```python
from build123d import *

# Parameters (mm, degrees)
EXTRUDE010_DEPTH = 5
SKETCH010_R      = 2
EXTRUDE009_DEPTH = 5
SKETCH012_R      = 2.1
EXTRUDE011_DEPTH = 5


with BuildPart() as extrude010:
    # Sketch011 (on Face6 of Extrude009) → Extrude010 (new body)
    with BuildSketch(Plane(origin=(0, 64.406042, 20.6), x_dir=(-1, 0, 0), z_dir=(0, 1, 0))):
        with BuildLine():
            Line((-18.188271, 0), (-18.188271, 36.810456))
            ThreePointArc((-12.998727, 42), (-16.668289, 40.480018), (-18.188271, 36.810456))
            Line((-12.998727, 42), (37.622185, 42))
            ThreePointArc((42.811729, 36.810456), (41.291746, 40.480018), (37.622185, 42))
            Line((42.811729, 0), (42.811729, 36.810456))
            Line((-18.188271, 0), (42.811729, 0))
        make_face()
        with BuildLine():
            Line((-9.188271, 5), (-9.188271, 33.276052))
            ThreePointArc((-5.464323, 37), (-8.097552, 35.909281), (-9.188271, 33.276052))
            Line((-5.464323, 37), (30.08778, 37))
            ThreePointArc((33.811729, 33.276052), (32.721009, 35.909281), (30.08778, 37))
            Line((33.811729, 33.276052), (33.811729, 5))
            Line((-9.188271, 5), (33.811729, 5))
        make_face(mode=Mode.SUBTRACT)
    extrude(amount=-EXTRUDE010_DEPTH)


with BuildPart() as extrude009:
    # Sketch010 → Extrude009 (new body)
    with BuildSketch(Plane.XY):
        Polygon((11.188271, 48.406042), (11.188271, 59.406042), (-35.811729, 59.406042), (-35.811729, 48.406042), (-42.811729, 48.406042), (-42.811729, 64.406042), (18.188271, 64.406042), (18.188271, 48.406042), align=None)
        with Locations((-39.061729, 52.906042)):
            Circle(SKETCH010_R, mode=Mode.SUBTRACT)
        with Locations((14.438271, 52.906042)):
            Circle(SKETCH010_R, mode=Mode.SUBTRACT)
    extrude(amount=EXTRUDE009_DEPTH)


with BuildPart() as extrude009_1:
    # Extrude009 placement: moved
    add(extrude009.part.moved(Location((0, 0, 20.6))))


with BuildPart() as pcb_holder_fusion:
    # Sketch012 (on Face3 of Extrude010) → Extrude011 (new body)
    with BuildSketch(Plane.XY.offset(62.6)):
        with BuildLine():
            Line((-37.622185, 64.406042), (-37.622185, 58.771772))
            ThreePointArc((-37.622185, 58.771772), (-36.898048, 57.023553), (-35.149829, 56.299416))
            Line((-35.149829, 56.299416), (10.526371, 56.299416))
            ThreePointArc((10.526371, 56.299416), (12.274591, 57.023553), (12.998727, 58.771772))
            Line((12.998727, 64.406042), (12.998727, 58.771772))
            Line((-37.622185, 64.406042), (12.998727, 64.406042))
        make_face()
        with Locations((-27.801273, 59.699416)):
            Circle(SKETCH012_R, mode=Mode.SUBTRACT)
        with Locations((3.198727, 59.799416)):
            Circle(SKETCH012_R, mode=Mode.SUBTRACT)
    extrude(amount=-EXTRUDE011_DEPTH)


with BuildPart() as pcb_holder_fusion_1:
    # Extrude011 placement: moved
    add(pcb_holder_fusion.part.moved(Location((0, -5, 0))))

    # Fusion012: union Extrude010, Extrude009
    add(extrude010.part)
    add(extrude009_1.part)


solid = pcb_holder_fusion_1.part
```
Work out the finished part from the listing and answer in its coordinate system (mm). A direction names the side the tool comes from. Round coordinates to 2 decimals unless told otherwise and drop trailing zeros. Order: outer loops, then holes, each group sorted by start corner. A loop starts at its lowest first (then second) coordinate and runs counter-clockwise, first axis right, second up.
Q1. A tool of negligible diameter and unlimited length cuts with its end or side. For faces 1 (the flat face through (9.188, 62, 40)), 2 (the flat face through (12.999, 57, 60)), 3 (the flat face through (-39.3, 55.2, 25.6)), from which of +Z, -Z, +X, -X, +Y, -Y can it reach the whole face along a straight path? Write none if from no direction.
Solution:
face 1: +Y, -Y
face 2: +Z, +X, -Y
face 3: +X, -X, -Y
Q2. Find the intervals of material crossed by line 1 along Z through (x, y) = (-13, 61); line 2 along X through (y, z) = (52, 23); line 3 along X through (y, z) = (61.5, 32.5), in increasing order.
Solution:
line 1: z = 20.6 to 25.6, 57.6 to 62.6
line 2: x = -42.81 to -40.84, -37.28 to -35.81, 11.19 to 12.66, 16.22 to 18.19
line 3: x = -42.81 to -33.81, 9.19 to 18.19
Q3. Given pin 1 Ø3.5 at (x, y) = (15.5, 55.5) entering from +Z; pin 2 Ø2.5 at (x, z) = (-18, 60.5) entering from -Y; pin 3 Ø2.5 at (y, z) = (56, 60) entering from +X, each flat-ended and moving along its own axis, determine where each tip first touches the part or whether it passes through.
Solution:
pin 1: stops at z = 25.6
pin 2: stops at y = 51.3
pin 3: stops at x = 13
Q4. A cutting plane is placed at A-A, the plane y = 49.5. Determine the outline of the cut face in (x, z), then the cut area to 3 significant figures.
Solution:
outline: (-42.81, 20.6) - (-35.81, 20.6) - (-35.81, 25.6) - (-42.81, 25.6) - close; (11.19, 20.6) - (18.19, 20.6) - (18.19, 25.6) - (11.19, 25.6) - close
area: 70.0 mm2
Q5. The mould has two halves that part along Z. Classify faces 4 (the flat face through (-33.812, 62, 40)), 5 (the flat face through (-12, 58, 62.6)), 6 (the flat face through (-37.622, 57, 60)): pulls with the +Z half, pulls with the -Z half, needs draft (parallel to the pull), parting line crosses it, or undercut.
Solution:
face 4: undercut
face 5: pulls with the +Z half
face 6: needs draft
Q6. A cutting plane is placed at C-C, the plane y = 61.5. Determine the outline of the cut face in (x, z), then the cut area to 3 significant figures.
Solution:
outline: (-42.81, 20.6) - (18.19, 20.6) - (18.19, 57.41) arc R5.19 ccw to (13, 62.6) - (-37.62, 62.6) arc R5.19 ccw to (-42.81, 57.41) - close; hole (-33.81, 25.6) - (9.19, 25.6) - (9.19, 53.88) arc R3.72 ccw to (5.46, 57.6) - (-30.09, 57.6) arc R3.72 ccw to (-33.81, 53.88) - close
area: 1,180 mm2
Q7. A cutting plane is placed at B-B, the plane z = 44.5. Determine the outline of the cut face in (x, y).
Solution:
outline: (-42.81, 59.41) - (-33.81, 59.41) - (-33.81, 64.41) - (-42.81, 64.41) - close; (9.19, 59.41) - (18.19, 59.41) - (18.19, 64.41) - (9.19, 64.41) - close
Q8. A cutting plane is placed at D-D, the plane x = -27.5. Determine the outline of the cut face in (y, z), then the cut area to 3 significant figures.
Solution:
outline: (51.3, 57.6) - (52.62, 57.6) - (52.62, 62.6) - (51.3, 62.6) - close; (56.78, 57.6) - (64.41, 57.6) - (64.41, 62.6) - (56.78, 62.6) - close; (59.41, 20.6) - (64.41, 20.6) - (64.41, 25.6) - (59.41, 25.6) - close
area: 69.8 mm2
